```python
from build123d import *

# Parameters (mm, degrees)
F1_DEPTH = 12.7
F3_DEPTH = 63.5
F4_R     = 6.3025
F5_DEPTH = 92.896292


with BuildPart() as f1:
    # F0 (on Front) → F1 (new body)
    with BuildSketch(Plane.XZ):
        Polygon((-93.092211, 0), (0, 0), (-41.521776, 61.619077), (-93.092211, 61.619077), align=None)
    extrude(amount=F1_DEPTH)

    # F2 (on face) → F3 (join)
    with BuildSketch(Plane.XZ.offset(12.7)):
        Polygon((-92.895292, 51.001634), (-92.895292, 0), (-8.06691, 0), (-46.175938, 51.001634), align=None)
    extrude(amount=F3_DEPTH)

    # F4 (on face) → F5 (cut, through all)
    with BuildSketch(Plane(origin=(-92.895292, 0, 0), x_dir=(0, -1, 0), z_dir=(-1, 0, 0))):
        with Locations((42.469766, 25.216423)):
            Circle(F4_R)
    extrude(amount=-F5_DEPTH, mode=Mode.SUBTRACT)


solid = f1.part
```
Could you check a few things on this model? Use its own coordinates, in mm. A direction names the side the tool comes from. Coordinates: 2 decimals unless noted, no trailing zeros. Order: outer loops, then holes, each group sorted by start corner. A loop starts at its lowest first (then second) coordinate and runs counter-clockwise, first axis right, second up. Notation, with made-up numbers: M 24.5,47.5 L 62.5,47.5 A23 ccw 62.5,71.5 Z; hole C 17,29 d9. An arc over 180 degrees is marked long. Use one line per item in the form item = value. Start each with the question number.
1. Please list where these lines run through material, in increasing order: line 1 (Z direction, x = -74, y = -70.5); line 2 (Y direction, x = -57, z = 26); line 3 (Y direction, x = -63, z = 59.5).
2. On a 3-axis mill with a long thin cutter (end or side, diameter ignored), from which of +Z, -Z, +X, -X, +Y, -Y can I reach the whole of each face in a straight line? I mean faces 1 (the flat face through (-20.47, -6.26, 30.38)), 2 (the flat face through (-92.895, -44, 32)), 3 (the flat face through (-69, -44, 51.002)). Say none if no direction works.
3. Suppose I cut it at C-C on z = 33.5. Write out the boundary of the cut face in (x, y).
4. We'd pull the mould along Z, two halves only. Please class faces 4 (the flat face through (-61, -76.2, 26)), 5 (the cylindrical face through (-57.987, -45.378, 19.625)), 6 (the flat face through (-26.85, -51.06, 25.14)), 7 (the flat face through (-47, -38, 0)): +Z half, -Z half, draft (parallel to the pull), parting line (faces both ways), or undercut.
5. For pin 1 (1.5 mm diameter, centred on y = -53.5, z = 47.5, fed in from -X); pin 2 (10 mm diameter, centred on x = -36, z = 21, fed in from +Y); pin 3 (1 mm diameter, centred on x = -58.5, y = -25, fed in from +Z), each with a flat end and sliding along its axis, tell me the tip position at first contact or that it passes through.
6. Suppose I cut it at D-D on y = -69. Write out the boundary of the cut face in (x, z), then the cut area to 3 significant figures.
7. Suppose I cut it at A-A on y = -46. Write out the boundary of the cut face in (x, z), then the cut area to 3 significant figures.
8. Suppose I cut it at B-B on x = -43. Write out the boundary of the cut face in (y, z) (1 decimal).
Geometry says:
q1.line_1 = 0 to 51
q1.line_2 = -76.2 to -48.72, -36.22 to 0
q1.line_3 = -12.7 to 0
q2.face_1 = +Z, +X, +Y, -Y
q2.face_2 = +Z, -Z, -X, -Y
q2.face_3 = +Z, +X, -X, -Y
q3.outline = M -93.09,-12.7 L -92.9,-12.7 L -92.9,-76.2 L -33.1,-76.2 L -33.1,-12.7 L -22.57,-12.7 L -22.57,0 L -93.09,0 Z
q4.face_4 = draft
q4.face_5 = undercut
q4.face_6 = +Z half
q4.face_7 = -Z half
q5.pin_1 = -92.9
q5.pin_2 = 0
q5.pin_3 = 51
q6.outline = M -92.9,0 L -8.07,0 L -46.18,51 L -92.9,51 Z
q6.area = 3,350 mm^2
q7.outline = M -92.9,0 L -8.07,0 L -23.01,20 L -92.9,20 Z; M -92.9,30.44 L -30.81,30.44 L -46.18,51 L -92.9,51 Z
q7.area = 2,670 mm^2
q8.outline = M -76.2,0 L 0,0 L 0,61.6 L -12.7,61.6 L -12.7,46.8 L -76.2,46.8 Z; hole C -42.5,25.2 d12.6
